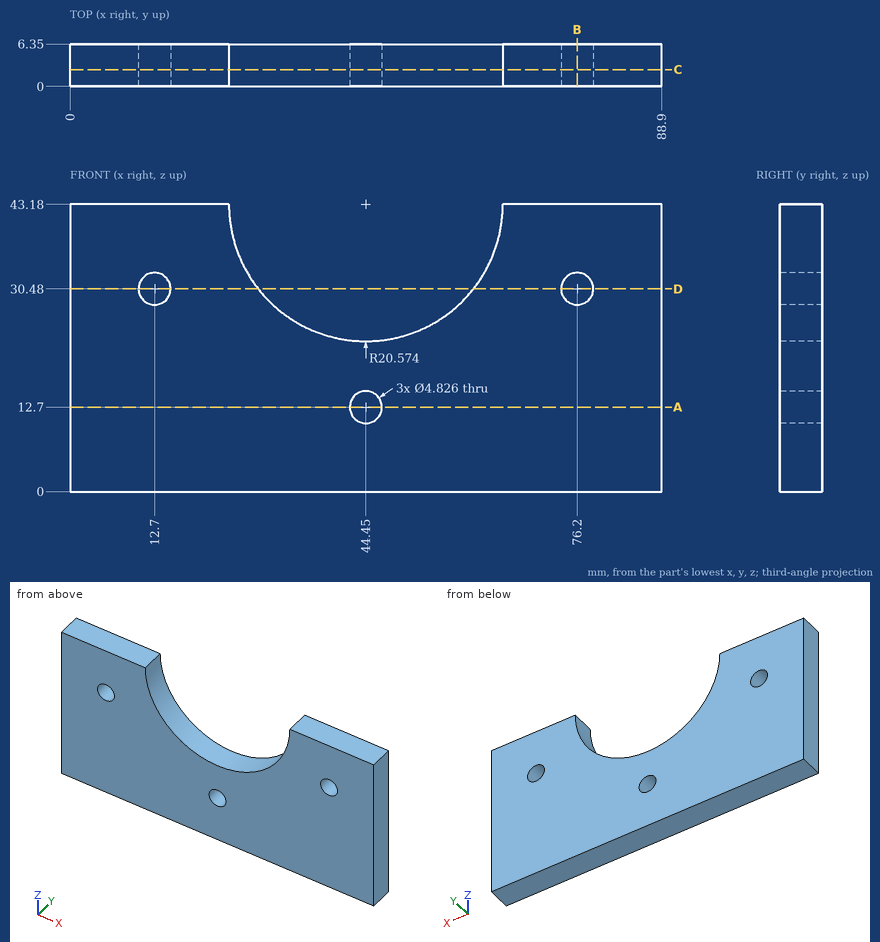
Here's the drawing with two shaded views (mm, measured from the low corner). I have some questions. Give positions to 0.01 mm unless a question says otherwise; leave off trailing zeros. Loops run counter-clockwise (first coordinate to the right, second up) from the corner with the lowest first, then second, coordinate; pieces in that order, holes last. Notation, with made-up numbers: M 74.25,20 L 120.25,20 A26 ccw 120.25,36 Z; hole C -11.5,-4.5 d2. An arc over 180 degrees is marked long. Answer in a Markdown table with one row per item.
1. Suppose I cut it at C-C on y = 2.5. Write out the boundary of the cut face in (x, z), plus the area to 3 significant figures.
Taken from the geometry:
| item | result |
|---|---|
| outline | M 0,0 L 88.9,0 L 88.9,43.18 L 65.02,43.18 A20.57 cw 23.88,43.18 L 0,43.18 Z; hole C 12.7,30.48 d4.83; hole C 44.45,12.7 d4.83; hole C 76.2,30.48 d4.83 |
| area | 3,120 mm² |
2. For pin 1 Ø8 at (x, z) = (53.5, 6) entering from -Y, with a flat end and sliding along its axis, tell me the tip position at first contact or that it passes through.
Taken from the geometry:
| item | result |
|---|---|
| pin 1 | stops at y = 0 |
3. Suppose I cut it at A-A on z = 12.7. Write out the boundary of the cut face in (x, y), plus the area to 3 significant figures.
Taken from the geometry:
| item | result |
|---|---|
| outline | M 0,0 L 42.04,0 L 42.04,6.35 L 0,6.35 Z; M 46.86,0 L 88.9,0 L 88.9,6.35 L 46.86,6.35 Z |
| area | 534 mm² |
4. Suppose I cut it at B-B on x = 76.2. Write out the boundary of the cut face in (y, z), plus the area to 3 significant figures.
Taken from the geometry:
| item | result |
|---|---|
| outline | M 0,0 L 6.35,0 L 6.35,28.07 L 0,28.07 Z; M 0,32.89 L 6.35,32.89 L 6.35,43.18 L 0,43.18 Z |
| area | 244 mm² |
5. Suppose I cut it at D-D on z = 30.48. Write out the boundary of the cut face in (x, y).
Taken from the geometry:
| item | result |
|---|---|
| outline | M 0,0 L 10.29,0 L 10.29,6.35 L 0,6.35 Z; M 15.11,0 L 28.26,0 L 28.26,6.35 L 15.11,6.35 Z; M 60.64,0 L 73.79,0 L 73.79,6.35 L 60.64,6.35 Z; M 78.61,0 L 88.9,0 L 88.9,6.35 L 78.61,6.35 Z |
6. If I drill on line 1 along Z through (x, y) = (44.45, 4.75); line 2 along X through (y, z) = (3.5, 30.48); line 3 along X through (y, z) = (1.5, 12.5), over which ranges is the centre line in solid material (lowest first)?
Taken from the geometry:
| item | result |
|---|---|
| line 1 | z = 0 to 10.29, 15.11 to 22.61 |
| line 2 | x = 0 to 10.29, 15.11 to 28.26, 60.64 to 73.79, 78.61 to 88.9 |
| line 3 | x = 0 to 42.05, 46.85 to 88.9 |
